Can you work these out from the drawing? Everything is in mm from the part's minimum corner. A direction names the side the tool comes from. Give positions to 0.01 mm unless a question says otherwise; leave off trailing zeros. Loops run counter-clockwise (first coordinate to the right, second up) from the corner with the lowest first, then second, coordinate; pieces in that order, holes last. Notation, with made-up numbers: M 36,-39.75 L 95,-39.75 A20 ccw 95,-7.75 Z; hole C -29,-13.75 d11. An arc over 180 degrees is marked long. Use CSV: the item, a comma, the result in double quotes.
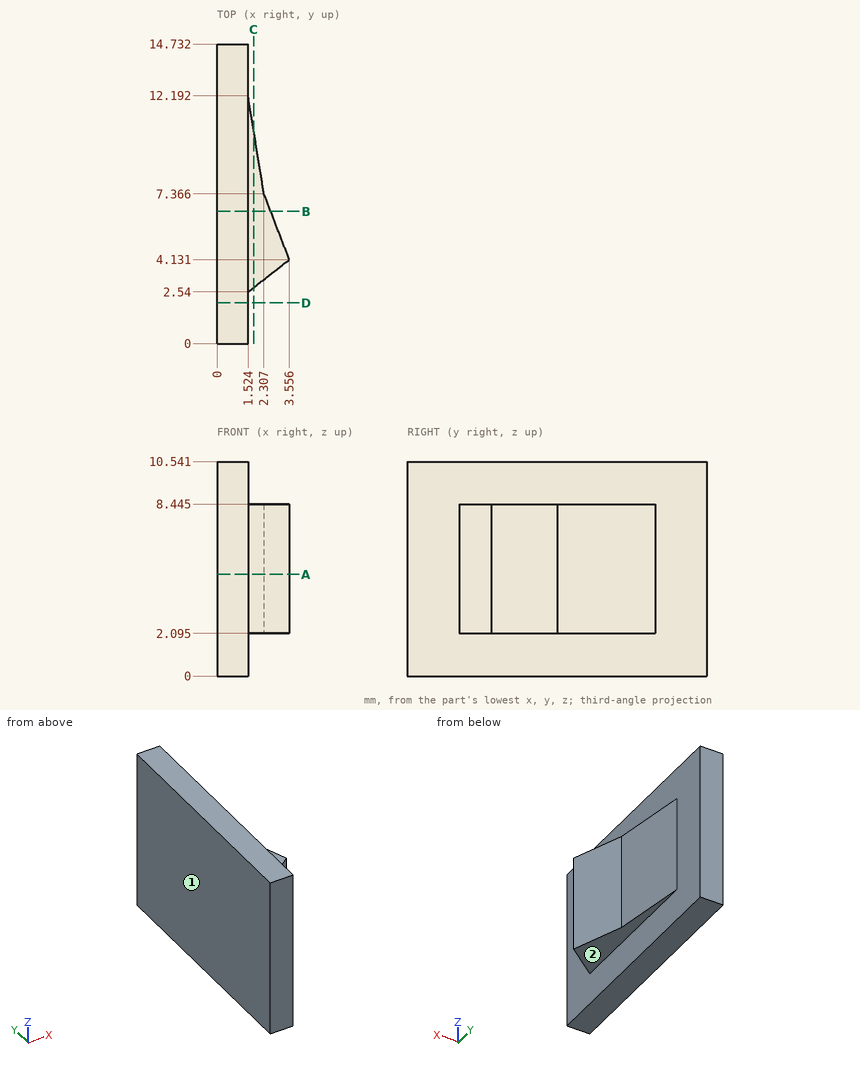
Q1. I want a section at A-A, the plane z = 5. Please give me the cut outline in (x, y) (1 decimal).
Model answer:
outline,"M 0,0 L 1.5,0 L 1.5,2.5 L 3.6,4.1 L 2.3,7.4 L 1.5,12.2 L 1.5,14.7 L 0,14.7 Z"
Q2. Please list where these lines run through material, in increasing order: L1, parallel to X at y = 13.25, z = 8 (1 decimal); L2, parallel to Z at x = 1.75, y = 6.5 (1 decimal); L3, parallel to X at y = 6.5, z = 3.5. Write a range as from..to.
Model answer:
L1,"0..1.5"
L2,"2.1..8.4"
L3,"0..2.64"
Q3. I'm going to push flat-ended pins straight in: P1, Ø1.6, axis at x = 2.5, y = 5, coming from the +Z side (1 decimal); P2, Ø0.6, axis at x = 2.5, y = 9, coming from the -Z side; P3, Ø3, axis at y = 10, z = 5, coming from the +X side. Where does each tip first touch, or does it pass through?
Model answer:
P1,"z = 8.4"
P2,"through"
P3,"x = 2.12"
Q4. I want a section at B-B, the plane y = 6.5. Please give me the cut outline in (x, z) (1 decimal).
Model answer:
outline,"M 0,0 L 1.5,0 L 1.5,2.1 L 2.6,2.1 L 2.6,8.4 L 1.5,8.4 L 1.5,10.5 L 0,10.5 Z"
Q5. I want a section at D-D, the plane y = 2. Please give me the cut outline in (x, z) (1 decimal).
Model answer:
outline,"M 0,0 L 1.5,0 L 1.5,10.5 L 0,10.5 Z"
Q6. For the marked faces 1 and 2, which set-ups out of +Z, -Z, +X, -X, +Y, -Y let a thin tool reach every point of the face, with its end or its side?
Model answer:
face 1,"+Z, -Z, -X, +Y, -Y"
face 2,"-Z, +X, +Y, -Y"
Q7. I want a section at C-C, the plane x = 1.8. Please give me the cut outline in (y, z) (1 decimal).
Model answer:
outline,"M 2.8,2.1 L 10.5,2.1 L 10.5,8.4 L 2.8,8.4 Z"
